Can you work these out from the drawing? Everything is in mm from the part's minimum corner. A direction names the side the tool comes from. Give positions to 0.01 mm unless a question says otherwise; leave off trailing zeros. Write each loop counter-clockwise with the first axis right and the second up, starting at its lowest first coordinate (ties: lowest second). Pieces come first, ordered by that corner, then holes. Notation, with made-up numbers: (-24, 72.5) - (7, 72.5) arc R21 ccw to (7, 96.5) - close; hole circle Ø2 at (-9, -34). An arc over 180 degrees is marked (long way). Write each question's results on one line, items separated by ' | '. Start each with the question number.
Item 1: Which directions (+Z, -Z, +X, -X, +Y, -Y) give clear straight access to the entire face, cutting with the end or side of a thin tool? Please do the marked faces 4, 5 and 6.
Item 2: Will these pins go through, and if not, where does the flat tip stop? P1, Ø1, axis at x = 77, z = 7.5, coming from the +Y side; P2, Ø3, axis at y = 36, z = 36.5, coming from the -X side; P3, Ø15, axis at x = 6.5, z = 17.5, coming from the +Y side.
Item 3: Suppose I cut it at A-A on y = 19.05. Count the separate pieces of the cut face and the enclosed holes in it.
Item 4: Please list where these lines run through material, in increasing order: line 1 along Z through (x, y) = (57.5, 15.5); line 2 along Y through (x, z) = (90, 10.5).
Item 5: Suppose I cut it at C-C on x = 37. List the corners of the cut face in (y, z) for me.
Item 6: We'd pull the mould along Z, two halves only. Please class the marked faces 1, 2 and 3: +Z half, -Z half, draft (parallel to the pull), parting line (faces both ways), or undercut.
Item 7: Suppose I cut it at B-B on x = 27. List the corners of the cut face in (y, z) for me.
Item 8: Suppose I cut it at D-D on z = 17.5. List the corners of the cut face in (x, y) for me.
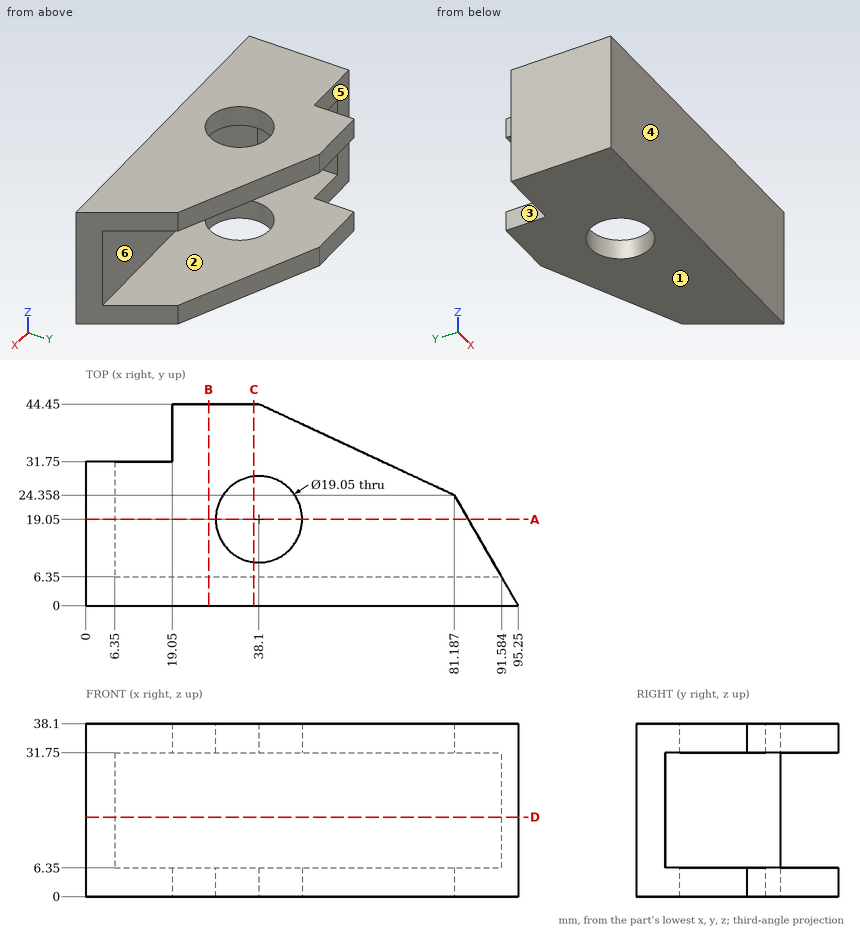
Checked values:
1) face 4: +Z, -Z, +X, -X, -Y | face 5: +Z, -Z, -X, +Y | face 6: +X, +Y
2) P1: stops at y = 6.35 | P2: stops at x = 19.05 | P3: stops at y = 31.75
3) separate pieces: 3 | enclosed holes: 0
4) line 1: z = 0 to 6.35, 31.75 to 38.1 | line 2: y = 0 to 6.35
5) outline: (0, 0) - (9.59, 0) - (9.59, 6.35) - (6.35, 6.35) - (6.35, 31.75) - (9.59, 31.75) - (9.59, 38.1) - (0, 38.1) - close; (28.51, 0) - (44.45, 0) - (44.45, 6.35) - (28.51, 6.35) - close; (28.51, 31.75) - (44.45, 31.75) - (44.45, 38.1) - (28.51, 38.1) - close
6) face 1: -Z half | face 2: undercut | face 3: draft
7) outline: (0, 0) - (44.45, 0) - (44.45, 6.35) - (6.35, 6.35) - (6.35, 31.75) - (44.45, 31.75) - (44.45, 38.1) - (0, 38.1) - close
8) outline: (0, 0) - (95.25, 0) - (91.58, 6.35) - (6.35, 6.35) - (6.35, 31.75) - (0, 31.75) - close
